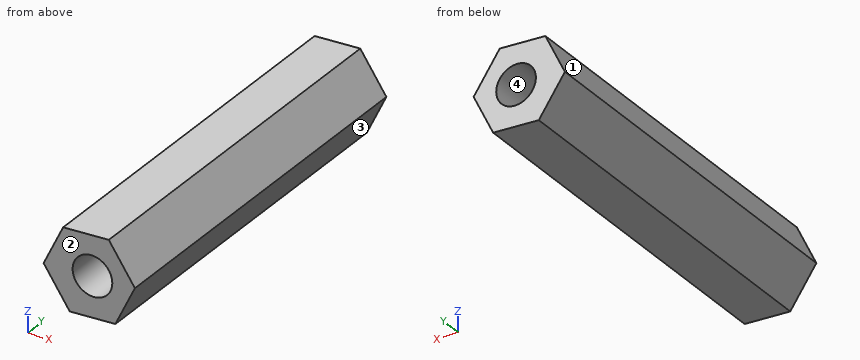
Autodesk Inventor part; units mm, degrees
ref_plane "YZ Plane" through (0, 0, 0) normal (1, 0, 0) x (0, 1, 0)
ref_plane "XZ Plane" through (0, 0, 0) normal (0, 1, 0) x (-1, 0, 0)
ref_plane "XY Plane" through (0, 0, 0) normal (0, 0, 1) x (1, 0, 0)
sketch "Sketch1" plane through (0, 0, 0) normal (0, 1, 0) x (-1, 0, 0)
  line L0 (-8.2612, 21.3942) -> (-12.4421, 15.3706)
  line L1 (-12.4421, 15.3706) -> (-19.7491, 15.9795)
  line L2 (-19.7491, 15.9795) -> (-22.8753, 22.612)
  line L3 (-22.8753, 22.612) -> (-18.6944, 28.6356)
  line L4 (-18.6944, 28.6356) -> (-11.3874, 28.0267)
  line L5 (-11.3874, 28.0267) -> (-8.2612, 21.3942)
  point P0 (0, 0)
  point P1 (-15.5682, 22.0031)
  dimension "d0" = 12.7
extrude "Extrusion1" add sketch "Sketch1" along normal blind 58.42
sketch "Sketch4" plane through (0, 58.42, 0) normal (0, 1, 0) x (1, 0, 0)
  circle A0 centre (16.0831, -22.124) radius 3.175
  point P0 (0, 0)
  dimension "d4" = 6.35
extrude "Extrusion2" cut sketch "Sketch4" against normal through all
properties part number "Hex Shaft"
For this review, take the finished solid that the model builds, in its own axes (mm). Face numbers are marked on the shaded views. Coordinates: 2 decimals unless noted, no trailing zeros. Loops run counter-clockwise (first coordinate to the right, second up) from the corner with the lowest first, then second, coordinate; pieces in that order, holes last. Notation, with made-up numbers: (7.5, 50) - (54.5, 50) arc R23 cw to (54.5, 86) - close; hole circle Ø2 at (-39, -7.5). An arc over 180 degrees is marked (long way). Return JSON: item names as keys, results as strings.
Item 1: Mouldability with a two-part tool opening along Z and no side actions: class the marked faces 1, 2, 3 and 4 as pulls with the +Z half, pulls with the -Z half, needs draft (parallel to the pull), parting line crosses it, or undercut.
Determined:
{"face 1": "pulls with the +Z half", "face 2": "needs draft", "face 3": "pulls with the -Z half", "face 4": "undercut"}
Item 2: Insertion check: pin 1 (5 mm diameter, centred on x = 14.5, y = 44, fed in from +Z); pin 2 (3 mm diameter, centred on x = 13, y = 33.5, fed in from +Z); pin 3 (5 mm diameter, centred on x = 19, y = 45.5, fed in from -Z). Each pin has a flat end and moves straight along its axis. Give the tip position at first contact, or say it passes through.
Determined:
{"pin 1": "stops at z = 28.49", "pin 2": "stops at z = 28.29", "pin 3": "stops at z = 15.71"}
Item 3: Take a section at D-D (z = 17.5). Give the boundary of the cut face in (x, y).
Determined:
{"outline": "(10.96, 0) - (20.47, 0) - (20.47, 58.42) - (10.96, 58.42) - close"}
Item 4: Take a section at A-A (z = 24). Give the boundary of the cut face in (x, y), then the cut area to 3 significant figures.
Determined:
{"outline": "(9.49, 0) - (13.52, 0) - (13.52, 58.42) - (9.49, 58.42) - close; (18.64, 0) - (21.91, 0) - (21.91, 58.42) - (18.64, 58.42) - close", "area": "426 mm2"}
Item 5: For line 1 (Z direction, x = 18.5, y = 19); line 2 (X direction, y = 54.5, z = 24.75); line 3 (X direction, y = 40, z = 20.75), list the stretches that pass through material, from the lowest coordinate up.
Determined:
{"line 1": "z = 15.88 to 20.07, 24.18 to 28.62", "line 2": "x = 9.84 to 14.3, 17.87 to 21.39", "line 3": "x = 8.71 to 13.22, 18.95 to 22"}
Item 6: Take a section at B-B (x = 14.25). Give the boundary of the cut face in (y, z).
Determined:
{"outline": "(0, 15.52) - (58.42, 15.52) - (58.42, 19.53) - (0, 19.53) - close; (0, 24.72) - (58.42, 24.72) - (58.42, 28.27) - (0, 28.27) - close"}
